Geometry: final body of the model. Coordinates: model frame, mm. A direction names the side the tool comes from. Give positions to 0.01 mm unless a question says otherwise; leave off trailing zeros. Write each loop counter-clockwise with the first axis right and the second up, starting at its lowest first coordinate (ties: lowest second). Pieces come first, ordered by that corner, then holes. Notation, with made-up numbers: (60.25, 71.25) -> (96.25, 71.25) arc R13 cw to (96.25, 79.25) -> close; hole circle Ø10 at (59.25, -30.5). An arc over 180 degrees is marked (long way). Answer in a Markdown table with one row per item. Add a question column.
Item 1: Draft query along Z for faces 1 (the conical face through (-65.18, -38.71, 0.4)), 2 (the flat face through (-59, 36, 22)), 3 (the flat face through (59, 8, 20.5)). Return one class per face: +Z half, -Z half, draft (parallel to the pull), parting line (faces both ways), or undercut.
Item 2: Section query D-D on z = 7. Output: boundary loops of the cut face in (x, y), plus the area to 3 significant figures.
Item 3: Material intervals for probe 1 along Y at (x, z) = (4, 9); probe 2 along X at (y, z) = (7, 18.75); probe 3 along X at (y, z) = (-0.5, 3.75), sorted ascending. Write a range as from..to.
Item 4: Access query for faces 4 (the flat face through (-1, 30, 2)), 5 (the flat face through (-1, -23, 12)), 6 (the flat face through (-50, 7, 7)). Directions: +Z, -Z, +X, -X, +Y, -Y. A direction counts if a zero-diameter tool reaches every point of the face in a straight line with its end or side. Return the directions, or none.
Item 5: Section query A-A on y = 2. Output: boundary loops of the cut face in (x, z).
Item 6: Section query C-C on x = 16. Output: boundary loops of the cut face in (y, z).
Item 7: First-contact query: P1, Ø1.2, axis at x = 3.5, z = 11, coming from the +Y side; P2, Ø2.5, axis at x = 55, z = 17, coming from the -Y side; P3, Ø2, axis at y = 48.5, z = 19, coming from the -X side. Flat tips, straight axial feed; report the tip coordinate or a pass-through.
```python
from build123d import *

# Parameters (mm, degrees)
SKETCH_W             = 133
SKETCH_H             = 90
PAD_DEPTH            = 10
PAD001_DEPTH         = 24
PAD002_DEPTH         = 133
SKETCH003_W          = 101
SKETCH003_H          = 2
PAD003_DEPTH         = 14
SKETCH004_W          = 100
SKETCH004_H          = 55
POCKET_DEPTH         = 6
SKETCH005_W          = 90
SKETCH005_H          = 45
POCKET001_DEPTH      = 24.001
FILLET_R             = 3
FILLET001_R          = 3
CHAMFER_SIZE         = 1
SKETCH006_W          = 6
SKETCH006_H          = 6
POCKET002_DEPTH      = 57
POCKET002_DEPTH_BACK = -57
SKETCH007_W          = 3.5
SKETCH007_H          = 57
POCKET003_DEPTH      = 3.5


with BuildPart() as part:
    # Sketch → Pad (new body)
    with BuildSketch(Plane.XY):
        with Locations((0, 5)):
            Rectangle(SKETCH_W, SKETCH_H)
    extrude(amount=PAD_DEPTH)

    # Sketch001 → Pad001 (join)
    with BuildSketch(Plane.XY):
        with BuildLine():
            Line((-66.5, -40), (-66.5, 50))
            Line((-66.5, 50), (-54, 50))
            Line((-54, 50), (-54, 48))
            Line((-54, 48), (-57, 48))
            Line((-57, 48), (-57, 42))
            Line((-57, 42), (-54, 42))
            Line((-54, 42), (-54, 40))
            Line((-54, 40), (-57, 40))
            Line((-57, 40), (-57, -32))
            Line((-57, -32), (-55.06066, -33.93934))
            ThreePointArc((-55.06066, -36.06066), (-54.62132, -35), (-55.06066, -33.93934))
            Line((-55.06066, -36.06066), (-57, -38))
            Line((-57, -38), (-57, -40))
            Line((-57, -40), (-66.5, -40))
        make_face()
    pad001 = extrude(amount=PAD001_DEPTH)

    # Mirrored: Pad001 across Sketch001 V_Axis
    add(pad001.mirror(Plane(origin=(0, 0, 0), x_dir=(0, 0, 1), z_dir=(1, 0, 0))))

    # Sketch002 (on Face10 of Mirrored) → Pad002 (join)
    with BuildSketch(Plane(origin=(-66.5, 0, 0), x_dir=(0, -1, 0), z_dir=(-1, 0, 0))):
        with BuildLine():
            Line((32, 10), (33.93934, 11.93934))
            ThreePointArc((36.06066, 11.93934), (35, 12.37868), (33.93934, 11.93934))
            Line((36.06066, 11.93934), (38, 10))
            Line((38, 10), (32, 10))
        make_face()
    extrude(amount=-PAD002_DEPTH)

    # Sketch003 → Pad003 (join)
    with BuildSketch(Plane.XY):
        with Locations((0, -24)):
            Rectangle(SKETCH003_W, SKETCH003_H)
    extrude(amount=PAD003_DEPTH)

    # Sketch004 (on Face32 of Pad003) → Pocket (cut)
    with BuildSketch(Plane.XY.offset(10)):
        with Locations((0, 7.5)):
            Rectangle(SKETCH004_W, SKETCH004_H)
    extrude(amount=-POCKET_DEPTH, mode=Mode.SUBTRACT)

    # Sketch005 → Pocket001 (cut, through all)
    with BuildSketch(Plane.XY):
        with Locations((0, 7.5)):
            Rectangle(SKETCH005_W, SKETCH005_H)
    extrude(amount=POCKET001_DEPTH, mode=Mode.SUBTRACT)

    # Fillet
    fillet_edges = [part.edges().sort_by_distance(p)[0] for p in [
        (66.5, 50, 5),
        (66.5, 50, 17),
        (66.5, -40, 5),
        (66.5, -40, 17),
    ]]
    fillet(fillet_edges, radius=FILLET_R)

    # Fillet001
    fillet001_edges = [part.edges().sort_by_distance(p)[0] for p in [
        (-66.5, -40, 17),
        (-66.5, -40, 5),
        (-66.5, 50, 17),
        (-66.5, 50, 5),
    ]]
    fillet(fillet001_edges, radius=FILLET001_R)

    # Chamfer
    chamfer_edges = [part.edges().sort_by_distance(p)[0] for p in [
        (0, 50, 0),
        (-58.75, 50, 0),
        (-65.62132, 49.12132, 0),
        (-66.5, 5, 0),
        (-65.62132, -39.12132, 0),
        (-60.25, -40, 0),
        (0, -40, 0),
        (60.25, -40, 0),
        (65.62132, -39.12132, 0),
        (66.5, 5, 0),
        (65.62132, 49.12132, 0),
        (58.75, 50, 0),
    ]]
    chamfer(chamfer_edges, length=CHAMFER_SIZE)

    # Sketch006 → Pocket002 (cut, two sides)
    with BuildSketch(Plane.YZ) as pocket002_sk:
        with Locations((45, 8)):
            Rectangle(SKETCH006_W, SKETCH006_H)
    extrude(amount=-POCKET002_DEPTH, mode=Mode.SUBTRACT)
    extrude(pocket002_sk.sketch, amount=-POCKET002_DEPTH_BACK, mode=Mode.SUBTRACT)

    # Sketch007 (on Face59 of Pocket002) → Pocket003 (cut)
    with BuildSketch(Plane.XY.offset(24)):
        with Locations((58.75, 7.5)):
            Rectangle(SKETCH007_W, SKETCH007_H)
        with Locations((-58.75, 7.5)):
            Rectangle(SKETCH007_W, SKETCH007_H)
    extrude(amount=-POCKET003_DEPTH, mode=Mode.SUBTRACT)


solid = part.part
```
Findings below:
| question | item | result |
|---|---|---|
| 1 | face 1 | -Z half |
| 1 | face 2 | draft |
| 1 | face 3 | +Z half |
| 2 | outline | (-66.5, -37) arc R3 ccw to (-63.5, -40) -> (63.5, -40) arc R3 ccw to (66.5, -37) -> (66.5, 47) arc R3 ccw to (63.5, 50) -> (-63.5, 50) arc R3 ccw to (-66.5, 47) -> close; hole (-57, 42) -> (57, 42) -> (57, 48) -> (-57, 48) -> close; hole (-50, -20) -> (50, -20) -> (50, 35) -> (-50, 35) -> close |
| 2 | area | 5,780 mm^2 |
| 3 | probe 1 | y = -40..-20, 35..42, 48..50 |
| 3 | probe 2 | x = -66.5..-57, 57..66.5 |
| 3 | probe 3 | x = -66.5..-45, 45..66.5 |
| 4 | face 4 | +Z, -Z |
| 4 | face 5 | +Z, +Y |
| 4 | face 6 | +Z |
| 5 | outline | (-66.5, 1) -> (-65.5, 0) -> (-45, 0) -> (-45, 4) -> (-50, 4) -> (-50, 10) -> (-57, 10) -> (-57, 20.5) -> (-60.5, 20.5) -> (-60.5, 24) -> (-66.5, 24) -> close; (45, 0) -> (65.5, 0) -> (66.5, 1) -> (66.5, 24) -> (60.5, 24) -> (60.5, 20.5) -> (57, 20.5) -> (57, 10) -> (50, 10) -> (50, 4) -> (45, 4) -> close |
| 6 | outline | (-40, 1) -> (-39, 0) -> (-15, 0) -> (-15, 4) -> (-20, 4) -> (-20, 10) -> (-23, 10) -> (-23, 14) -> (-25, 14) -> (-25, 10) -> (-32, 10) -> (-33.94, 11.94) arc R1.5 ccw to (-36.06, 11.94) -> (-38, 10) -> (-40, 10) -> close; (30, 0) -> (49, 0) -> (50, 1) -> (50, 10) -> (48, 10) -> (48, 5) -> (42, 5) -> (42, 10) -> (35, 10) -> (35, 4) -> (30, 4) -> close |
| 7 | P1 | stops at y = -23 |
| 7 | P2 | stops at y = -37.25 |
| 7 | P3 | stops at x = -66.46 |
